Check sheet for the modelled part. Datum: model origin and axes. Units: mm. Face numbers are marked on the shaded views. A direction names the side the tool comes from. Coordinates: 2 decimals unless noted, no trailing zeros. Write each loop counter-clockwise with the first axis right and the second up, starting at its lowest first coordinate (ties: lowest second). Pieces come first, ordered by that corner, then holes. Notation, with made-up numbers: (81, 79) -> (136, 79) arc R18 ccw to (136, 114) -> close; hole circle Ø1 at (45.25, -38.5). An arc over 180 degrees is marked (long way). One line per item, written item: value. Start each with the question number.
1) Gauge pin test, flat ends, axial feed: P1, Ø10, axis at x = 42, z = 3, coming from the +Y side; P2, Ø4, axis at x = 37, z = 5, coming from the +Y side (3 decimals); P3, Ø1.5, axis at y = -4, z = 12, coming from the -X side; P4, Ø6.5, axis at x = -11, y = 9.5, coming from the -Z side. Record the tip position at first contact, or that the pin passes through.
2) Sectioned sample at A-A on x = -4. Enter the section's corners in (y, z) (3 decimals), plus the area to 3 significant figures.
3) Draft check along Z on the marked faces 3, 4 and 5. Enter one of: +Z half, -Z half, draft (parallel to the pull), parting line (faces both ways), or undercut.
4) Sectioned sample at D-D on x = 60.5. Enter the section's corners in (y, z).
5) Scan lines: line 1 along Z through (x, y) = (43, -8.25); line 2 along Z through (x, y) = (4.5, 2.25); line 3 along Y through (x, z) = (-28, 33). Record each from-to range of solid material in increasing order. Write a range as [from, to].
6) Sectioned sample at B-B on z = 48. Enter the section's corners in (x, y) (3 decimals), plus the area to 3 significant figures.
7) Sectioned sample at C-C on y = 6. Enter the section's corners in (x, z), plus the area to 3 significant figures.
8) Set-up check for the marked faces 1 and 2: record each of +Z, -Z, +X, -X, +Y, -Y from which the full face is reachable in a straight line by a thin tool's end or side.
```python
from build123d import *

# Parameters (mm, degrees)
F1_DEPTH = 12.7
F0_W     = 4.2696557939
F0_H     = 24.5932303369
F2_DEPTH = 4.445
F3_DEPTH = 4.445
F4_DEPTH = 13.97


with BuildPart() as f1:
    # F0 (on Front) → F1 (new body, symmetric)
    with BuildSketch(Plane.XZ):
        Polygon((-60.8683489263, 37.8787778318), (-65.1380047202, 37.8787778318), (-65.1380047202, 25.7041221485), (35.7967093587, 25.7041221485), (35.7967093587, 37.8787778318), align=None)
        Polygon((35.7967093587, 25.7041221485), (-65.1380047202, 25.7041221485), (-65.1380047202, 13.5294664651), (-60.8683489263, 13.5294664651), (35.7967093587, 13.5294664651), align=None)
    extrude(amount=F1_DEPTH, both=True)

    # F0 (on Front) → F2 (join)
    with BuildSketch(Plane.XZ):
        with Locations((-63.0031768233, 50.1753930002)):
            Rectangle(F0_W, F0_H)
        with Locations((-63.0031768233, 1.2328512967)):
            Rectangle(F0_W, F0_H)
    extrude(amount=-F2_DEPTH)

    # F0 (on Front) → F3 (join, symmetric)
    with BuildSketch(Plane.XZ):
        Polygon((33.7472744286, 62.4720081687), (-60.8683489263, 62.4720081687), (-60.8683489263, 37.8787778318), (35.7967093587, 37.8787778318), (37.7412438393, 37.8787778318), (52.0139420338, 49.3214614689), (33.7472744286, 49.3214614689), align=None)
        with BuildLine():
            ThreePointArc((5.5675311014, 52.4003553908), (8.6464250233, 49.3214614689), (5.5675311014, 46.2425675471))
            Line((5.5675311014, 46.2425675471), (-29.1020926088, 46.2425675471))
            ThreePointArc((-29.1020926088, 46.2425675471), (-32.1809865307, 49.3214614689), (-29.1020926088, 52.4003553908))
            Line((-29.1020926088, 52.4003553908), (5.5675311014, 52.4003553908))
        make_face(mode=Mode.SUBTRACT)
        Polygon((37.7412438393, 13.5294664651), (35.7967093587, 13.5294664651), (-60.8683489263, 13.5294664651), (-60.8683489263, -11.0637638718), (33.7472744286, -11.0637638718), (33.7472744286, 2.086782828), (52.0139420338, 2.086782828), align=None)
        with BuildLine():
            ThreePointArc((-29.1020926088, -3.0788939219), (-32.1809865307, 0), (-29.1020926088, 3.0788939219))
            Line((-29.1020926088, 3.0788939219), (5.5675311014, 3.0788939219))
            ThreePointArc((5.5675311014, 3.0788939219), (8.6464250233, 0), (5.5675311014, -3.0788939219))
            Line((5.5675311014, -3.0788939219), (-29.1020926088, -3.0788939219))
        make_face(mode=Mode.SUBTRACT)
    extrude(amount=F3_DEPTH, both=True)

    # F0 (on Front) → F4 (join, symmetric)
    with BuildSketch(Plane.XZ):
        Polygon((68.4168934822, 62.4720081687), (33.7472744286, 62.4720081687), (33.7472744286, 49.3214614689), (52.0139420338, 49.3214614689), align=None)
        Polygon((68.4168934822, -11.0637638718), (52.0139420338, 2.086782828), (33.7472744286, 2.086782828), (33.7472744286, -11.0637638718), align=None)
    extrude(amount=F4_DEPTH, both=True)


solid = f1.part
```
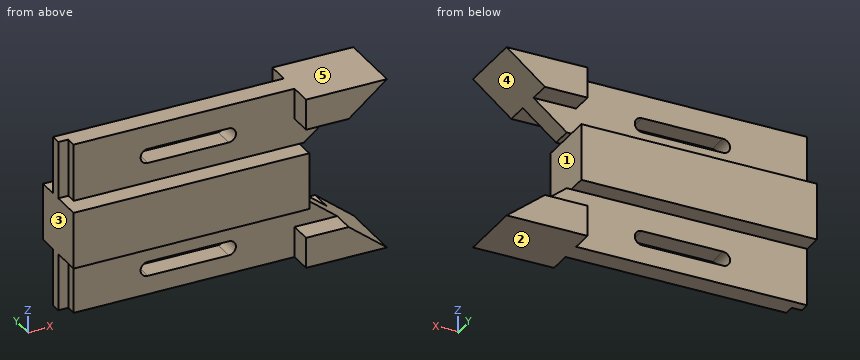
Answers:
1. P1: stops at y = 13.97
1. P2: stops at y = 4.445
1. P3: stops at x = -60.87
1. P4: stops at z = 13.53
2. outline: (-12.7, 13.529) -> (-4.445, 13.529) -> (-4.445, 3.079) -> (4.445, 3.079) -> (4.445, 13.529) -> (12.7, 13.529) -> (12.7, 37.879) -> (4.445, 37.879) -> (4.445, 46.243) -> (-4.445, 46.243) -> (-4.445, 37.879) -> (-12.7, 37.879) -> close; (-4.445, -11.064) -> (4.445, -11.064) -> (4.445, -3.079) -> (-4.445, -3.079) -> close; (-4.445, 52.4) -> (4.445, 52.4) -> (4.445, 62.472) -> (-4.445, 62.472) -> close
2. area: 946 mm2
3. face 3: draft
3. face 4: undercut
3. face 5: +Z half
4. outline: (-13.97, -11.06) -> (13.97, -11.06) -> (13.97, -4.72) -> (-13.97, -4.72) -> close; (-13.97, 56.12) -> (13.97, 56.12) -> (13.97, 62.47) -> (-13.97, 62.47) -> close
5. line 1: z = [-11.06, 2.09], [49.32, 62.47]
5. line 2: z = [-11.06, -3.08], [3.08, 46.24], [52.4, 62.47]
5. line 3: y = [-12.7, 12.7]
6. outline: (-65.138, 0) -> (-60.868, 0) -> (-60.868, -4.445) -> (-31.883, -4.445) -> (-31.883, 4.445) -> (-65.138, 4.445) -> close; (8.348, -4.445) -> (50.366, -4.445) -> (50.366, 4.445) -> (8.348, 4.445) -> close
6. area: 650 mm2
7. outline: (-65.14, 13.53) -> (35.8, 13.53) -> (35.8, 37.88) -> (-65.14, 37.88) -> close; (33.75, -11.06) -> (68.42, -11.06) -> (52.01, 2.09) -> (33.75, 2.09) -> close; (33.75, 49.32) -> (52.01, 49.32) -> (68.42, 62.47) -> (33.75, 62.47) -> close
7. area: 3,150 mm2
8. face 1: +X, +Y, -Y
8. face 2: -Z, +X, -X, +Y, -Y
